CAD build for the part. Positions are in the model's coordinates, mm. Give positions to 0.01 mm unless a question says otherwise; leave off trailing zeros. Loops run counter-clockwise (first coordinate to the right, second up) from the corner with the lowest first, then second, coordinate; pieces in that order, holes last. Notation, with made-up numbers: M 34.5,79 L 90.5,79 A31 ccw 90.5,108 Z; hole C 62.5,-36 d3. An arc over 180 degrees is marked long. Answer as CSV lines item,"result".
```python
from build123d import *

# Parameters (mm, degrees)
SKETCH_1_R          = 1.65
SKETCH_1_R_2        = 7.5
EXTRUDE_1_DEPTH     = 5
CUT_EXTRUDE_1_DEPTH = 5
CUT_EXTRUDE_3_DEPTH = 5


with BuildPart() as part:
    # 草图1 → 凸台-拉伸1 (new body)
    with BuildSketch(Plane(origin=(0, 0, 0), x_dir=(1, 0, 0), z_dir=(0, 1, 0))):
        with BuildLine():
            Line((120, 0), (125, 0))
            ThreePointArc((125, 0), (132.071067812, -2.928932188), (135, -10))
            Line((135, -10), (135, -120.9))
            Line((135, -120.9), (150, -120.9))
            Line((150, -120.9), (150, -180.9))
            Line((150, -180.9), (135, -180.9))
            Line((135, -180.9), (135, -190))
            ThreePointArc((135, -190), (132.071067812, -197.071067812), (125, -200))
            Line((125, -200), (89.5, -200))
            Line((89.5, -200), (89.5, -189.35))
            ThreePointArc((89.5, -189.35), (89.207106781, -188.642893219), (88.5, -188.35))
            Line((88.5, -188.35), (41.5, -188.35))
            ThreePointArc((41.5, -188.35), (40.792893219, -188.642893219), (40.5, -189.35))
            Line((40.5, -189.35), (40.5, -200))
            Line((40.5, -200), (5, -200))
            ThreePointArc((5, -200), (-2.071067812, -197.071067812), (-5, -190))
            Line((-5, -190), (-5, -10))
            ThreePointArc((-5, -10), (-2.071067812, -2.928932188), (5, 0))
            Line((5, 0), (10, 0))
            Line((10, 0), (120, 0))
        make_face()
        with Locations(Location((19, -10, 0), (0, 0, 270))):
            Circle(SKETCH_1_R, mode=Mode.SUBTRACT)
        with Locations(Location((111, -10, 0), (0, 0, 270))):
            Circle(SKETCH_1_R, mode=Mode.SUBTRACT)
        with Locations(Location((15, -25, 0), (0, 0, 270))):
            Circle(SKETCH_1_R_2, mode=Mode.SUBTRACT)
        with Locations(Location((115, -25, 0), (0, 0, 90))):
            Circle(SKETCH_1_R_2, mode=Mode.SUBTRACT)
        with Locations(Location((-0.4, -45.5, 0), (0, 0, 270))):
            Circle(SKETCH_1_R, mode=Mode.SUBTRACT)
        with Locations(Location((51.6, -45.5, 0), (0, 0, 270))):
            Circle(SKETCH_1_R, mode=Mode.SUBTRACT)
        with Locations(Location((51.6, -124.1, 0), (0, 0, 270))):
            Circle(SKETCH_1_R, mode=Mode.SUBTRACT)
        with Locations(Location((-0.4, -124.1, 0), (0, 0, 270))):
            Circle(SKETCH_1_R, mode=Mode.SUBTRACT)
        with Locations(Location((89.5, -45.6, 0), (0, 0, 270))):
            Circle(SKETCH_1_R, mode=Mode.SUBTRACT)
        with Locations(Location((131.5, -45.6, 0), (0, 0, 270))):
            Circle(SKETCH_1_R, mode=Mode.SUBTRACT)
        with Locations(Location((131.5, -113.8, 0), (0, 0, 270))):
            Circle(SKETCH_1_R, mode=Mode.SUBTRACT)
        with Locations(Location((89.5, -113.8, 0), (0, 0, 270))):
            Circle(SKETCH_1_R, mode=Mode.SUBTRACT)
        with Locations(Location((146, -128, 0), (0, 0, 270))):
            Circle(SKETCH_1_R, mode=Mode.SUBTRACT)
        with Locations(Location((100, -128, 0), (0, 0, 270))):
            Circle(SKETCH_1_R, mode=Mode.SUBTRACT)
        with Locations(Location((100, -174, 0), (0, 0, 270))):
            Circle(SKETCH_1_R, mode=Mode.SUBTRACT)
        with Locations(Location((146, -174, 0), (0, 0, 270))):
            Circle(SKETCH_1_R, mode=Mode.SUBTRACT)
        with Locations(Location((65, -155, 0), (0, 0, 270))):
            Circle(SKETCH_1_R_2, mode=Mode.SUBTRACT)
        with Locations(Location((96, -190, 0), (0, 0, 270))):
            Circle(SKETCH_1_R, mode=Mode.SUBTRACT)
        with Locations(Location((34, -190, 0), (0, 0, 90))):
            Circle(SKETCH_1_R, mode=Mode.SUBTRACT)
        with BuildLine():
            Line((96.35, -23.35), (96.35, -6.65))
            ThreePointArc((96.35, -6.65), (98, -5), (99.65, -6.65))
            Line((99.65, -6.65), (99.65, -23.35))
            ThreePointArc((99.65, -23.35), (98, -25), (96.35, -23.35))
        make_face(mode=Mode.SUBTRACT)
        with BuildLine():
            Line((30.35, -6.65), (30.35, -23.35))
            ThreePointArc((30.35, -23.35), (32, -25), (33.65, -23.35))
            Line((33.65, -23.35), (33.65, -6.65))
            ThreePointArc((33.65, -6.65), (32, -5), (30.35, -6.65))
        make_face(mode=Mode.SUBTRACT)
        with BuildLine():
            Line((17.85, -188.35), (12.15, -188.35))
            ThreePointArc((12.15, -188.35), (10.983273811, -188.833273811), (10.5, -190))
            ThreePointArc((10.5, -190), (10.983273811, -191.166726189), (12.15, -191.65))
            Line((12.15, -191.65), (17.85, -191.65))
            ThreePointArc((17.85, -191.65), (19.016726189, -191.166726189), (19.5, -190))
            ThreePointArc((19.5, -190), (19.016726189, -188.833273811), (17.85, -188.35))
        make_face(mode=Mode.SUBTRACT)
        with BuildLine():
            Line((112.15, -188.35), (117.85, -188.35))
            ThreePointArc((117.85, -188.35), (119.016726189, -188.833273811), (119.5, -190))
            ThreePointArc((119.5, -190), (119.016726189, -191.166726189), (117.85, -191.65))
            Line((117.85, -191.65), (112.15, -191.65))
            ThreePointArc((112.15, -191.65), (110.983273811, -191.166726189), (110.5, -190))
            ThreePointArc((110.5, -190), (110.983273811, -188.833273811), (112.15, -188.35))
        make_face(mode=Mode.SUBTRACT)
    extrude(amount=EXTRUDE_1_DEPTH)

    # 草图2 → 切除-拉伸1 (cut)
    with BuildSketch(Plane.XZ):
        with BuildLine():
            Line((42, 0), (88, 0))
            Line((88, 0), (88, 25))
            ThreePointArc((88, 25), (85.071067812, 32.071067812), (78, 35))
            Line((78, 35), (52, 35))
            ThreePointArc((52, 35), (44.928932188, 32.071067812), (42, 25))
            Line((42, 25), (42, 0))
        make_face()
    extrude(amount=-CUT_EXTRUDE_1_DEPTH, mode=Mode.SUBTRACT)

    # 草图4 → 切除-拉伸3 (cut)
    with BuildSketch(Plane(origin=(0, 0, 0), x_dir=(1, 0, 0), z_dir=(0, 1, 0))):
        with BuildLine():
            Line((75.25, -70), (75.25, -100))
            ThreePointArc((75.25, -100), (73.6, -101.65), (71.95, -100))
            Line((71.95, -100), (71.95, -70))
            ThreePointArc((71.95, -70), (73.6, -68.35), (75.25, -70))
        make_face()
    extrude(amount=CUT_EXTRUDE_3_DEPTH, mode=Mode.SUBTRACT)


solid = part.part
```
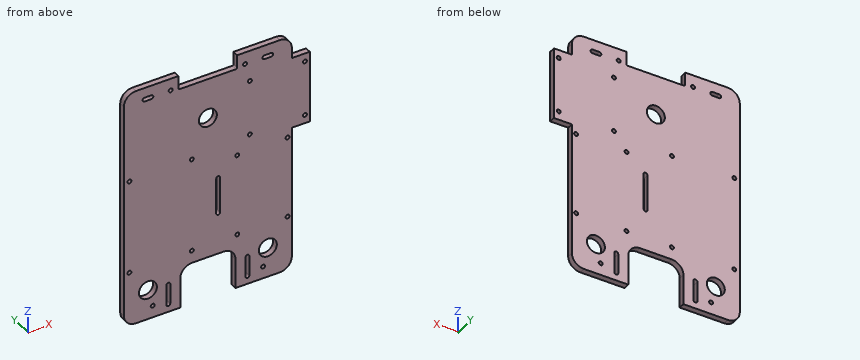
Q1. Cut at D-D (z = 40). Write the cut outline in (x, y), and give its area (3 significant figures).
Solution:
outline,"M -5,0 L 135,0 L 135,5 L -5,5 Z"
area,"700 mm²"
Q2. Wall check: line 1 (Z direction, x = 115, y = 3.2); line 2 (X direction, y = 1.5, z = 45.5); line 3 (X direction, y = 2.2, z = 10). Give the ranges that are in metal, low to high. Write a range as [from, to].
Solution:
line 1,"z = [0, 17.5], [32.5, 188.35], [191.65, 200]"
line 2,"x = [-5, -2.05], [1.25, 49.95], [53.25, 87.85], [91.15, 129.85], [133.15, 135]"
line 3,"x = [-5, 17.35], [20.65, 30.35], [33.65, 42], [88, 96.35], [99.65, 109.35], [112.65, 135]"
Q3. Pin check, flat tips, straight feed: P1, Ø2, axis at x = 146, z = 128, coming from the -Y side; P2, Ø2, axis at x = 47.5, y = 1.5, coming from the -Z side; P3, Ø3, axis at y = 1.5, z = 34.5, coming from the +X side. Stop position of each tip, or through.
Solution:
P1,"passes through"
P2,"stops at z = 33.35"
P3,"stops at x = 135"
Q4. Cut at A-A (z = 155). Write the cut outline in (x, y), and give its area (3 significant figures).
Solution:
outline,"M -5,0 L 57.5,0 L 57.5,5 L -5,5 Z; M 72.5,0 L 150,0 L 150,5 L 72.5,5 Z"
area,"700 mm²"
Q5. Cut at B-B (x = 15). Write the cut outline in (y, z).
Solution:
outline,"M 0,0 L 5,0 L 5,17.5 L 0,17.5 Z; M 0,32.5 L 5,32.5 L 5,188.35 L 0,188.35 Z; M 0,191.65 L 5,191.65 L 5,200 L 0,200 Z"
Q6. Cut at C-C (y = 2.55). Give the number of separate pieces and of enclosed holes in the cut face, and give its area (3 significant figures).
Solution:
separate pieces,"1"
enclosed holes,"24"
area,"25,700 mm²"
